```python
from build123d import *

# Parameters (mm, degrees)
EXTRUDE_1_DEPTH     = 3
SKETCH_2_R          = 1.1
SKETCH_2_R_2        = 1.025013192
SKETCH_2_R_3        = 1.6
CUT_EXTRUDE_2_DEPTH = 116.143388868
FILLET_1_R          = 5
SKETCH_3_R          = 1.6
SKETCH_3_R_2        = 1.1
EXTRUDE_2_DEPTH     = 3
CUT_EXTRUDE_3_DEPTH = 10
FILLET_2_R          = 3
EXTRUDE_3_DEPTH     = 3
SKETCH_6_W          = 3
SKETCH_6_H          = 59
EXTRUDE_4_DEPTH     = 2
SKETCH_7_W          = 102
SKETCH_7_H          = 3
EXTRUDE_5_DEPTH     = 1.7
FILLET_4_R          = 3


with BuildPart() as part:
    # 草图1 → 凸台-拉伸1 (new body)
    with BuildSketch(Plane.XY):
        Polygon((0, 0), (0, -57), (-42, -57), (-100, -5), (-100, 0), align=None)
    extrude(amount=EXTRUDE_1_DEPTH)

    # 草图2 → 切除-拉伸2 (cut, through all)
    with BuildSketch(Plane.XY.offset(3)):
        with Locations(Location((-38, -45, 0), (0, 0, 180))):
            Circle(SKETCH_2_R)
        with Locations(Location((-38, -14.5, 0), (0, 0, 180))):
            Circle(SKETCH_2_R)
        with Locations(Location((-38, -2.5, 0), (0, 0, 180))):
            Circle(SKETCH_2_R)
        with Locations(Location((-56, -2.5, 0), (0, 0, 180))):
            Circle(SKETCH_2_R)
        with Locations(Location((-74, -2.5, 0), (0, 0, 180))):
            Circle(SKETCH_2_R)
        with Locations(Location((-92, -2.5, 0), (0, 0, 180))):
            Circle(SKETCH_2_R)
        with Locations((-55.007781707, -42.651734732)):
            Circle(SKETCH_2_R_2)
        with Locations((-81.223203164, -24.300939713)):
            Circle(SKETCH_2_R_2)
        with Locations((-20, -2.5)):
            Circle(SKETCH_2_R)
        with Locations((-2, -2.5)):
            Circle(SKETCH_2_R)
        with Locations((-2, -14.5)):
            Circle(SKETCH_2_R)
        with Locations((-2, -45)):
            Circle(SKETCH_2_R)
        with Locations((-15, -54)):
            Circle(SKETCH_2_R_3)
        with Locations((-35, -54)):
            Circle(SKETCH_2_R_3)
    extrude(amount=-CUT_EXTRUDE_2_DEPTH, mode=Mode.SUBTRACT)

    # 圆角1
    fillet_1_edges = [part.edges().sort_by_distance(p)[0] for p in [
        (-100, -5, 1.5),
    ]]
    fillet(fillet_1_edges, radius=FILLET_1_R)

    # 草图3 → 凸台-拉伸2 (add)
    with BuildSketch(Plane.XY.offset(3)):
        with BuildLine():
            Line((-100, 0), (-100, -2.767468243))
            ThreePointArc((-100, -2.767468243), (-99.565557216, -4.806018538), (-98.337725079, -6.490315447))
            Line((-98.337725079, -6.490315447), (-42, -57))
            Line((-42, -57), (0, -57))
            Line((0, -57), (0, 0))
            Line((0, 0), (-100, 0))
        make_face()
        with Locations((-15, -54)):
            Circle(SKETCH_3_R, mode=Mode.SUBTRACT)
        with Locations((-35, -54)):
            Circle(SKETCH_3_R, mode=Mode.SUBTRACT)
        with Locations((-2, -2.5)):
            Circle(SKETCH_3_R_2, mode=Mode.SUBTRACT)
        with Locations((-20, -2.5)):
            Circle(SKETCH_3_R_2, mode=Mode.SUBTRACT)
        with Locations(Location((-38, -2.5, 0), (0, 0, 180))):
            Circle(SKETCH_3_R_2, mode=Mode.SUBTRACT)
        with Locations(Location((-56, -2.5, 0), (0, 0, 180))):
            Circle(SKETCH_3_R_2, mode=Mode.SUBTRACT)
        with Locations(Location((-74, -2.5, 0), (0, 0, 180))):
            Circle(SKETCH_3_R_2, mode=Mode.SUBTRACT)
        with Locations(Location((-92, -2.5, 0), (0, 0, 180))):
            Circle(SKETCH_3_R_2, mode=Mode.SUBTRACT)
    extrude(amount=-EXTRUDE_2_DEPTH)

    # 草图4 → 切除-拉伸3 (cut)
    with BuildSketch(Plane.XY.offset(3)):
        Polygon((-79.442813774, -10), (-42.214341741, -43.377250788), (-49.442813774, -10), align=None)
        Polygon((-33, -8), (-8, -18), (-24.986953422, -45), align=None)
    extrude(amount=-CUT_EXTRUDE_3_DEPTH, mode=Mode.SUBTRACT)

    # 圆角2
    fillet_2_edges = [part.edges().sort_by_distance(p)[0] for p in [
        (-79.442813774, -10, 1.5),
        (-49.442813774, -10, 1.5),
        (-42.214341741, -43.377250788, 1.5),
        (-24.986953422, -45, 1.5),
        (-33, -8, 1.5),
        (-8, -18, 1.5),
    ]]
    fillet(fillet_2_edges, radius=FILLET_2_R)

    # 草图5 → 凸台-拉伸3 (add)
    with BuildSketch(Plane.XY.offset(3)):
        Polygon((0, -57), (-42, -57), (-39.769230769, -59), (0, -59), align=None)
    extrude(amount=-EXTRUDE_3_DEPTH)

    # 草图6 → 凸台-拉伸4 (add)
    with BuildSketch(Plane(origin=(0, 0, 0), x_dir=(0, 0, -1), z_dir=(1, 0, 0))):
        with Locations((-1.5, -29.5)):
            Rectangle(SKETCH_6_W, SKETCH_6_H)
    extrude(amount=EXTRUDE_4_DEPTH)

    # 草图7 → 凸台-拉伸5 (add)
    with BuildSketch(Plane(origin=(0, 0, 0), x_dir=(1, 0, 0), z_dir=(0, 1, 0))):
        with Locations((-49, -1.5)):
            Rectangle(SKETCH_7_W, SKETCH_7_H)
    extrude(amount=EXTRUDE_5_DEPTH)

    # 圆角4
    fillet_4_edges = [part.edges().sort_by_distance(p)[0] for p in [
        (-39.769230769, -59, 1.5),
        (2, -59, 1.5),
        (2, 1.7, 1.5),
        (-100, 1.7, 1.5),
    ]]
    fillet(fillet_4_edges, radius=FILLET_4_R)


solid = part.part
```
For this review, take the finished solid that the model builds, in its own axes (mm). A direction names the side the tool comes from. Coordinates: 2 decimals unless noted, no trailing zeros. Write each loop counter-clockwise with the first axis right and the second up, starting at its lowest first coordinate (ties: lowest second). Pieces come first, ordered by that corner, then holes.
(1) Add section A-A on x = -35. Give the boundary of the cut face in (y, z), then the cut area to 4 significant figures.
(2) For pin 1 Ø1.3 at (x, y) = (-74, -2.5) entering from -Z; pin 2 Ø1.5 at (x, z) = (-57, 1) entering from -Y, all flat-tipped, find the tip position at first contact; note any pin that passes through.
(3) Add section B-B on z = 0.5. Count the separate pieces of the cut face and the enclosed holes in it, then the cut area to 3 significant figures.
(4) Add section D-D on x = -56. Give the boundary of the cut face in (y, z), then the cut area to 3 significant figures.
(5) Tool access review of faces 1 (the face through (1.1, -58.14, 1.48)), 2 (the face through (-74.422, -11.975, 1.479)): name each direction out of +Z, -Z, +X, -X, +Y, -Y from which nothing blocks a thin tool from reaching the whole face with its end or side.
(6) The part is to be moulded in two halves that separate along Y. For faces 3 (the face through (-38, -29, 3)), 4 (the face through (-45.64, -37.58, 1.48)), 5 (the face through (-19.67, -13.33, 1.52)), 6 (the face through (-99.577, -4.779, 1.521)), say which applies: +Y half, -Y half, draft (parallel to the pull), parting line (faces both ways), or undercut.
(7) Add section C-C on y = -54. Give the boundary of the cut face in (x, z).
(8) Wall thickness on probe 1 along Y at (x, z) = (-38, 1); probe 2 along Y at (x, z) = (-74, 2.1); probe 3 along X at (y, z) = (-34.5, 2): over which ranges is each line inside the solid? List them lowest first.
Answer sheet:
1. outline: (-59, 0) - (-55.6, 0) - (-55.6, 3) - (-59, 3) - close; (-52.4, 0) - (1.7, 0) - (1.7, 3) - (-52.4, 3) - close
1. area: 172.5 mm2
2. pin 1: passes through
2. pin 2: stops at y = -44.22
3. separate pieces: 1
3. enclosed holes: 10
3. area: 3,650 mm2
4. outline: (-44.45, 0) - (-31.02, 0) - (-31.02, 3) - (-44.45, 3) - close; (-10, 0) - (-3.6, 0) - (-3.6, 3) - (-10, 3) - close; (-1.4, 0) - (1.7, 0) - (1.7, 3) - (-1.4, 3) - close
4. area: 68.8 mm2
5. face 1: +Z, -Z, +X, -Y
5. face 2: +Z, -Z
6. face 3: draft
6. face 4: undercut
6. face 5: undercut
6. face 6: -Y half
7. outline: (-45.35, 0) - (-36.6, 0) - (-36.6, 3) - (-45.35, 3) - close; (-33.4, 0) - (-16.6, 0) - (-16.6, 3) - (-33.4, 3) - close; (-13.4, 0) - (2, 0) - (2, 3) - (-13.4, 3) - close
8. probe 1: y = -59 to -3.6, -1.4 to 1.7
8. probe 2: y = -28.31 to -14.8, -11.2 to -3.6, -1.4 to 1.7
8. probe 3: x = -67.1 to -52.12, -44.14 to -27.26, -18.38 to 2
